Solid Edge part; units mm, degrees
sketch "Sketch1" plane through (0, 0, 0) normal (0, -1, 0) x (1, 0, 0)
  line L0 (-21.15, 17.15) -> (-21.15, -17.15)
  line L1 (-21.15, -17.15) -> (-17.15, -21.15)
  line L2 (-17.15, -21.15) -> (17.15, -21.15)
  line L3 (17.15, -21.15) -> (21.15, -17.15)
  line L4 (21.15, -17.15) -> (21.15, 17.15)
  line L5 (21.15, 17.15) -> (17.15, 21.15)
  line L6 (17.15, 21.15) -> (-17.15, 21.15)
  line L7 (-17.15, 21.15) -> (-21.15, 17.15)
  dimension "D1" = 17.15
extrude "Protrusion1" add sketch "Sketch1" along normal mid plane 35
sketch "Sketch2" plane through (0, 0, 0) normal (0, -1, 0) x (1, 0, 0)
  line L0 (-20.15, 16.3391) -> (-20.15, -16.3391)
  line L1 (-20.15, -16.3391) -> (-16.3391, -20.15)
  line L2 (-16.3391, -20.15) -> (16.3391, -20.15)
  line L3 (16.3391, -20.15) -> (20.15, -16.3391)
  line L4 (20.15, -16.3391) -> (20.15, 16.3391)
  line L5 (20.15, 16.3391) -> (16.3391, 20.15)
  line L6 (16.3391, 20.15) -> (-16.3391, 20.15)
  line L7 (-16.3391, 20.15) -> (-20.15, 16.3391)
extrude "ExtrudedCutout_1" cut sketch "Sketch2" along normal mid plane 25 flip side to cut
sketch "Sketch3" plane through (0, 0, 0) normal (1, 0, 0) x (0, 1, 0)
  line L0 (-17.5, 0) -> (-17.5, 11)
  line L1 (-17.5, 11) -> (-19.5, 11)
  line L2 (-19.5, 11) -> (-19.5, 2.5)
  line L3 (-19.5, 2.5) -> (-42.5, 2.5)
  line L4 (-42.5, 2.5) -> (-42.5, 0)
  dimension "D1" = 17.5
revolve "RevolvedProtrusion1" add sketch "Sketch3" angle 360 about axis through (0, -46, 0) along (0, 1, 0)
chamfer "Chamfer_1" distance 0.5 angle 45 2 edges at (0, -19.5, 11) (0, -42.5, 2.5)
hole "Hole_1" at (-15.5, -17.5, -15.5) direction (0, 1, 0) diameter 3.242 depth 4.5 tip angle 118 thread major 4 thread length 4
hole "Hole1" at (-15.5, -17.5, 15.5) direction (0, 1, 0) diameter 3.242 depth 4.5 tip angle 118 thread major 4 thread length 4
hole "Hole2" at (15.5, -17.5, -15.5) direction (0, 1, 0) diameter 3.242 depth 4.5 tip angle 118 thread major 4 thread length 4
hole "Hole3" at (15.5, -17.5, 15.5) direction (0, 1, 0) diameter 3.242 depth 4.5 tip angle 118 thread major 4 thread length 4
properties material "Stainless steel"
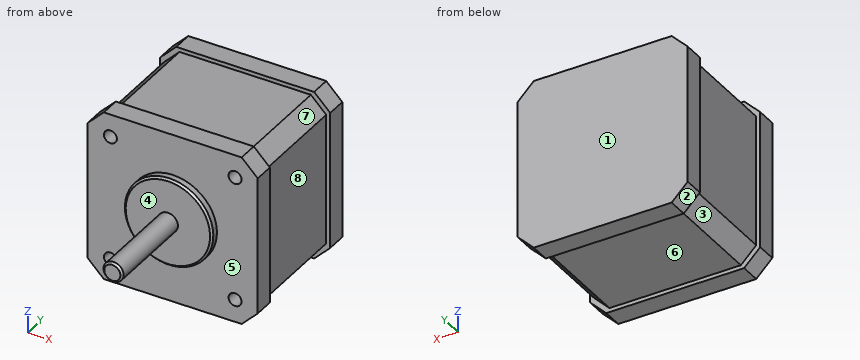
For this review, take the finished solid that the model builds, in its own axes (mm). Face numbers are marked on the shaded views. A direction names the side the tool comes from. Round coordinates to 2 decimals unless told otherwise and drop trailing zeros. Write each loop counter-clockwise with the first axis right and the second up, starting at its lowest first coordinate (ties: lowest second). Pieces come first, ordered by that corner, then holes. Notation, with made-up numbers: (42, 74.25) -> (51, 74.25) arc R31 cw to (51, 111.25) -> close; hole circle Ø4 at (-35, 80.5). An arc over 180 degrees is marked (long way). One line per question, with ' | ' between items. Start each with the question number.
(1) For line 1 along Z through (x, y) = (-15.5, -15.85); line 2 along X through (y, z) = (-14, -15), list the stretches that pass through material, from the lowest coordinate up. Write a range as from..to.
(2) Add section B-B, the plane z = 0. Write out the cut boundary in (x, y), plus the area to 3 significant figures.
(3) Add section A-A, the plane y = -15. Write out the cut boundary in (x, z), plus the area to 3 significant figures.
(4) Tool access review of the marked faces 5, 6, 7 and 8: name each direction out of +Z, -Z, +X, -X, +Y, -Y from which nothing blocks a thin tool from reaching the whole face with its end or side.
(5) Insertion check: P1, Ø7.5, axis at x = 2.5, y = -5.5, coming from the +Z side; P2, Ø12.5, axis at y = 2, z = -1, coming from the +X side; P3, Ø4, axis at y = 2, z = 4, coming from the -X side. Each pin has a flat end and moves straight along its axis. Give the tip position at first contact, or say it passes through.
(6) Add section D-D, the plane y = -21.5. Write out the cut boundary in (x, z), plus the area to 3 significant figures.
(7) Add section C-C, the plane x = -12.5. Write out the cut boundary in (y, z).
(8) Mouldability with a two-part tool opening along Y and no side actions: class the marked faces 1, 2, 3 and 4 as released by +Y, released by -Y, zero draft, split by the parting line, or undercut.
Answer list:
1) line 1: -21.15..-17.12, -13.88..13.88, 17.12..21.15 | line 2: -21.15..-17.04, -13.96..13.96, 17.04..21.15
2) outline: (-21.15, -17.5) -> (-11, -17.5) -> (-11, -19) -> (-10.5, -19.5) -> (-2.5, -19.5) -> (-2.5, -42) -> (-2, -42.5) -> (2, -42.5) -> (2.5, -42) -> (2.5, -19.5) -> (10.5, -19.5) -> (11, -19) -> (11, -17.5) -> (21.15, -17.5) -> (21.15, -12.5) -> (20.15, -12.5) -> (20.15, 12.5) -> (21.15, 12.5) -> (21.15, 17.5) -> (-21.15, 17.5) -> (-21.15, 12.5) -> (-20.15, 12.5) -> (-20.15, -12.5) -> (-21.15, -12.5) -> close | area: 1,590 mm²
3) outline: (-21.15, -17.15) -> (-17.15, -21.15) -> (17.15, -21.15) -> (21.15, -17.15) -> (21.15, 17.15) -> (17.15, 21.15) -> (-17.15, 21.15) -> (-21.15, 17.15) -> close; hole circle Ø3.24 at (-15.5, -15.5); hole circle Ø3.24 at (-15.5, 15.5); hole circle Ø3.24 at (15.5, -15.5); hole circle Ø3.24 at (15.5, 15.5) | area: 1,720 mm²
4) face 5: -Y | face 6: -Z, +X, -X | face 7: +Z, +X | face 8: +Z, -Z, +X
5) P1: z = 20.15 | P2: x = 20.15 | P3: x = -20.15
6) outline: circle Ø5 at (0, 0) | area: 19.6 mm²
7) outline: (-17.5, -21.15) -> (-12.5, -21.15) -> (-12.5, -20.15) -> (12.5, -20.15) -> (12.5, -21.15) -> (17.5, -21.15) -> (17.5, 21.15) -> (12.5, 21.15) -> (12.5, 20.15) -> (-12.5, 20.15) -> (-12.5, 21.15) -> (-17.5, 21.15) -> close
8) face 1: released by +Y | face 2: zero draft | face 3: undercut | face 4: released by -Y
